from build123d import *

# Parameters (mm, degrees)
SKETCH1_W           = 100
SKETCH1_H           = 45
BOSS_EXTRUDE1_DEPTH = 10
SKETCH3_W           = 31.4
SKETCH3_H           = 7.5
BOSS_EXTRUDE2_DEPTH = 5
SKETCH4_R           = 3.75
BOSS_EXTRUDE3_DEPTH = 7.5
CUT_EXTRUDE1_DEPTH  = 45
CUT_EXTRUDE2_DEPTH  = 100


with BuildPart() as part:
    # Sketch1 → Boss-Extrude1 (new body)
    with BuildSketch(Plane.XY):
        with Locations((26.050004349, -7.647768163)):
            Rectangle(SKETCH1_W, SKETCH1_H)
    extrude(amount=BOSS_EXTRUDE1_DEPTH)

    # Sketch3 → Boss-Extrude2 (add)
    with BuildSketch(Plane.XY.offset(10)):
        with Locations((1.750004349, 1.102231837)):
            Rectangle(SKETCH3_W, SKETCH3_H)
    boss_extrude2 = extrude(amount=BOSS_EXTRUDE2_DEPTH)

    # Sketch4 → Boss-Extrude3 (add)
    with BuildSketch(Plane.XZ.offset(2.647768163)):
        with BuildLine():
            Line((-13.949995651, 15), (-13.949995651, 27))
            ThreePointArc((-13.949995651, 27), (-9.556597369, 37.606601718), (1.050004349, 42))
            Line((1.050004349, 42), (2.450004349, 42))
            ThreePointArc((2.450004349, 42), (13.056606067, 37.606601718), (17.450004349, 27))
            Line((17.450004349, 27), (17.450004349, 15))
            Line((17.450004349, 15), (-13.949995651, 15))
        make_face()
        with Locations(Location((1.744890168, 27, 0), (0, 0, 270))):
            Circle(SKETCH4_R, mode=Mode.SUBTRACT)
    boss_extrude3 = extrude(amount=-BOSS_EXTRUDE3_DEPTH)

    # Mirror1: Boss-Extrude2, Boss-Extrude3 across plane
    add(boss_extrude2.mirror(Plane(origin=(0, -7.147768163, 0), x_dir=(0, 0, 1), z_dir=(0, -1, 0))))
    add(boss_extrude3.mirror(Plane(origin=(0, -7.147768163, 0), x_dir=(0, 0, 1), z_dir=(0, -1, 0))))

    # Sketch5 → Cut-Extrude1 (cut)
    with BuildSketch(Plane.XZ.offset(30.147768163)):
        Polygon((-13.949995651, 10), (-23.949995651, 7), (-23.949995651, 10), align=None)
        Polygon((17.450004349, 10), (76.050004349, 7), (76.050004349, 10), align=None)
    extrude(amount=-CUT_EXTRUDE1_DEPTH, mode=Mode.SUBTRACT)

    # Sketch6 → Cut-Extrude2 (cut)
    with BuildSketch(Plane.ZY.offset(23.949995651)):
        Polygon((7, 14.852231837), (10, 4.852231837), (10, 14.852231837), align=None)
        Polygon((10, -19.147768163), (7, -30.147768163), (10, -30.147768163), align=None)
    extrude(amount=-CUT_EXTRUDE2_DEPTH, mode=Mode.SUBTRACT)


solid = part.part
Build history of the part. All positions in model axes, mm. A direction names the side the tool comes from. Coordinates: 2 decimals unless noted, no trailing zeros. Order: outer loops, then holes, each group sorted by start corner. A loop starts at its lowest first (then second) coordinate and runs counter-clockwise, first axis right, second up. Notation, with made-up numbers: (65.25, 24.25) - (71.25, 24.25) arc R17 cw to (71.25, 47.25) - close; hole circle Ø5 at (-4.5, 13.5). An arc over 180 degrees is marked (long way). Put each result on its own line as item: value.
1. Saw through at C-C (y = -16.5). Write the cut outline in (x, z).
Answer sheet:
outline: (-23.95, 0) - (76.05, 0) - (76.05, 7) - (17.45, 10) - (17.45, 27) arc R15 ccw to (2.45, 42) - (1.05, 42) arc R15 ccw to (-13.95, 27) - (-13.95, 10) - (-23.95, 7) - close; hole circle Ø7.5 at (1.74, 27)
2. Saw through at D-D (y = 12.5). Write the cut outline in (x, z).
Answer sheet:
outline: (-23.95, 0) - (76.05, 0) - (76.05, 7) - (62.27, 7.71) - (-21.6, 7.71) - (-23.95, 7) - close
3. Probe line 1 along X through (y, z) = (-14, 27); line 2 along Y through (x, z) = (13.5, 18.5); line 3 along Z through (x, y) = (20.5, -15). List the from-to ranges inside material, lowest first. Write a range as [from, to].
Answer sheet:
line 1: x = [-13.95, -2.01], [5.49, 17.45]
line 2: y = [-19.15, -11.65], [-2.65, 4.85]
line 3: z = [0, 9.84]
4. Pull direction Z, two halves, no side cores. Call faces 1 (the face through (-1.916, 1.05, 27.813)), 2 (the face through (-9.67, -15.35, 37.49)), 3 (the face through (-23.95, -8, 3)): pulls with the +Z half, pulls with the -Z half, needs draft (parallel to the pull), parting line crosses it, or undercut.
Answer sheet:
face 1: undercut
face 2: pulls with the +Z half
face 3: needs draft
5. Tool access for faces 4 (the face through (17.45, -15, 19)), 5 (the face through (2, -7, 10)), 6 (the face through (2, 4.852, 23)), 7 (the face through (-13.95, 1, 18)): list every direction of +Z, -Z, +X, -X, +Y, -Y with a clear straight run to the whole face (end or side of a thin tool).
Answer sheet:
face 4: +Z, +X, +Y, -Y
face 5: +Z, +X, -X
face 6: +Z, +X, -X, +Y
face 7: +Z, -X, +Y, -Y
6. Drop flat-ended pins along their axis: P1, Ø2, axis at y = -5.5, z = 25.5, coming from the +X side; P2, Ø10, axis at x = 1.74, z = 27, coming from the -Y side; P3, Ø25, axis at x = 9.5, z = 30.5, coming from the +Y side; P4, Ø12, axis at y = -0.5, z = 25.5, coming from the +X side. Give the stop position or say it passes through.
Answer sheet:
P1: passes through
P2: stops at y = -19.15
P3: stops at y = 4.85
P4: stops at x = 17.45
7. Saw through at B-B (x = 15). Write the cut outline in (y, z).
Answer sheet:
outline: (-30.15, 0) - (14.85, 0) - (14.85, 7) - (4.85, 10) - (4.85, 35.22) - (-2.65, 35.22) - (-2.65, 10) - (-11.65, 10) - (-11.65, 35.22) - (-19.15, 35.22) - (-19.15, 10) - (-30.15, 7) - close
8. Saw through at A-A (z = 16). Write the cut outline in (x, y).
Answer sheet:
outline: (-13.95, -19.15) - (17.45, -19.15) - (17.45, -11.65) - (-13.95, -11.65) - close; (-13.95, -2.65) - (17.45, -2.65) - (17.45, 4.85) - (-13.95, 4.85) - close
